Source: CAD feature listing. Evaluate the final solid. Frame: model axes, mm. A direction names the side the tool comes from. Round coordinates to 2 decimals unless told otherwise and drop trailing zeros. Order: outer loops, then holes, each group sorted by start corner. A loop starts at its lowest first (then second) coordinate and runs counter-clockwise, first axis right, second up. Notation, with made-up numbers: (-28, -21.75) - (23, -21.75) arc R24 ccw to (23, 17.25) - close; hole circle Ø2 at (27.25, 24). An arc over 180 degrees is marked (long way). Return JSON: item names as keys, results as strings. Group by question number.
1) Ray query, line 1 (Z direction, x = 31.75, y = -105.25); line 2 (X direction, y = -24, z = 26); line 3 (Y direction, x = 59.5, z = 1). Return the intervals inside material, ascending. Write a range as from..to.
2) Mould query, pull axis Z, two halves, no side actions, for faces 5 (the flat face through (32, 25.4, -32)), 6 (the flat face through (6.35, 84, 30)), 7 (the flat face through (31.31, -70.54, -7.15)). Classes: pulls with the +Z half, pulls with the -Z half, needs draft (parallel to the pull), parting line crosses it, or undercut.
3) Section A-A, the plane x = 31.75. Give the number of separate pieces and of enclosed holes in the cut face, plus the area to 3 significant figures.
4) Access query for faces 1 (the flat face through (31.6, 55.1, 8.2)), 2 (the flat face through (50.8, -25, 16)), 3 (the flat face through (31.57, 43.85, -14.79)), 4 (the flat face through (9, 50.8, -41)). Directions: +Z, -Z, +X, -X, +Y, -Y. A direction counts if a zero-diameter tool reaches every point of the face in a straight line with its end or side. Return the directions, or none.
5) Section D-D, the plane z = 75. Return loops of the section in (x, y).
6) Section C-C, the plane y = 5. Return loops of the section in (x, z), plus the area to 3 significant figures.
7) Section B-B, the plane z = 8.5. Return loops of the section in (x, y), plus the area to 3 significant figures.
8) Contact query for flat-ended pins moving along their axis: P1, Ø24, axis at x = 17.5, z = 2.5, coming from the +Y side; P2, Ø4, axis at x = 59, y = -25, coming from the -Z side; P3, Ø6, axis at x = 46, z = 19, coming from the +Y side. Output: stop coordinate, or through.
```python
from build123d import *

# Parameters (mm, degrees)
F1_DEPTH  = 63.5
F2_W      = 25.4
F2_H      = 44.800144308
F3_DEPTH  = 25.4
F4_W      = 25.4
F4_H      = 31.5590774218
F5_DEPTH  = 25.4
F6_W      = 48.812078476
F6_H      = 72.883464396
F6_R      = 19.05
F7_DEPTH  = 25.4
F6_R_2    = 13.97
F8_DEPTH  = 90.17
F9_W      = 38.1
F9_H      = 50.8
F10_DEPTH = 33.02
F11_W     = 50.8
F11_H     = 61.1203222922
F12_DEPTH = 7.62
F13_R     = 2.54
F14_DEPTH = 584.2


with BuildPart() as f1:
    # F0 (on Right) → F1 (new body)
    with BuildSketch(Plane.YZ):
        Polygon((88.0636948228, -0.3382474043), (88.0636948228, 60.7820748879), (88.7095872307, 95.6336185336), (-34.4394557178, 95.6336185336), (-89.7363051772, 84.2712447047), (-89.7363051772, 0), (-50.8, -14.504159911), (-50.8, 0), (0, 0), (0, -20.0953550052), (50.8, -56.7663814664), (50.8, -25.2073040446), align=None)
        Polygon((72.5463054062, -2.1647087139), (72.4311518908, 1.9652569746), (75.9502303361, 4.1299656885), (79.5844622969, 2.1647087139), (79.6996158123, -1.9652569746), (76.1805373669, -4.1299656885), align=None, mode=Mode.SUBTRACT)
    extrude(amount=F1_DEPTH)

    # F2 (on face) → F3 (cut)
    with BuildSketch(Plane(origin=(0, 27.2928575232, -40.895508354), x_dir=(1, 0, 0), z_dir=(0, 0.5551110833, -0.831776223))):
        with Locations((31.75, -50.6614504268)):
            Rectangle(F2_W, F2_H)
    extrude(amount=-F3_DEPTH, mode=Mode.SUBTRACT)

    # F4 (on face) → F5 (cut)
    with BuildSketch(Plane(origin=(0, 50.8, 0), x_dir=(-1, 0, 0), z_dir=(0, 1, 0))):
        with Locations((-31.75, -40.9868427555)):
            Rectangle(F4_W, F4_H)
    extrude(amount=-F5_DEPTH, mode=Mode.SUBTRACT)

    # F6 (on face) → F7 (join)
    with BuildSketch(Plane.XZ.offset(89.7363051772)):
        with Locations((31.75, 42.1356223524)):
            Rectangle(F6_W, F6_H)
        with Locations((31.75, 42.1356223524)):
            Circle(F6_R, mode=Mode.SUBTRACT)
    extrude(amount=F7_DEPTH)

    # F6 (on face) → F8 (cut)
    with BuildSketch(Plane.XZ.offset(89.7363051772)):
        with Locations((31.75, 42.1356223524)):
            Circle(F6_R_2)
    extrude(amount=-F8_DEPTH, mode=Mode.SUBTRACT)

    # F9 (on face) → F10 (cut)
    with BuildSketch(Plane(origin=(0, 0, 0), x_dir=(1, 0, 0), z_dir=(0, 0, -1))):
        with Locations((31.75, 25.4)):
            Rectangle(F9_W, F9_H)
    extrude(amount=-F10_DEPTH, mode=Mode.SUBTRACT)

    # F11 (on face) → F12 (cut)
    with BuildSketch(Plane(origin=(0, 88.0636948228, 0), x_dir=(-1, 0, 0), z_dir=(0, 1, 0))):
        with Locations((-31.75, 30.2219137418)):
            Rectangle(F11_W, F11_H)
    extrude(amount=-F12_DEPTH, mode=Mode.SUBTRACT)

    # F13 (on face) → F14 (cut)
    with BuildSketch(Plane.XZ.offset(89.7363051772)):
        with Locations((31.7480713129, 42.1407744288)):
            Circle(F13_R)
    extrude(amount=-F14_DEPTH, mode=Mode.SUBTRACT)


solid = f1.part
```
Geometry check:
{
 "1": {"line 1": "5.69..23.09, 61.19..78.58", "line 2": "0..12.7, 50.8..63.5", "line 3": "-89.74..72.46, 79.62..88.06"},
 "2": {"face 5": "needs draft", "face 6": "undercut", "face 7": "pulls with the -Z half"},
 "3": {"separate pieces": "3", "enclosed holes": "0", "area": "13,800 mm2"},
 "4": {"face 1": "none", "face 2": "-Z", "face 3": "+Y", "face 4": "-Z, +X, -X, +Y"},
 "5": {"outline": "(0, -89.74) - (7.34, -89.74) - (7.34, -115.14) - (56.16, -115.14) - (56.16, -89.74) - (63.5, -89.74) - (63.5, 88.33) - (0, 88.33) - close"},
 "6": {"outline": "(0, -23.7) - (63.5, -23.7) - (63.5, 95.63) - (0, 95.63) - close; hole circle Ø5.08 at (31.75, 42.14)", "area": "7,560 mm2"},
 "7": {"outline": "(0, -89.74) - (7.34, -89.74) - (7.34, -115.14) - (56.16, -115.14) - (56.16, -89.74) - (63.5, -89.74) - (63.5, 88.06) - (57.15, 88.06) - (57.15, 80.44) - (44.45, 80.44) - (44.45, 55.55) - (19.05, 55.55) - (19.05, 80.44) - (6.35, 80.44) - (6.35, 88.06) - (0, 88.06) - close; hole (12.7, -50.8) - (50.8, -50.8) - (50.8, 0) - (12.7, 0) - close", "area": "9,580 mm2"},
 "8": {"P1": "y = 88.06", "P2": "z = 0", "P3": "y = 80.44"}
}
